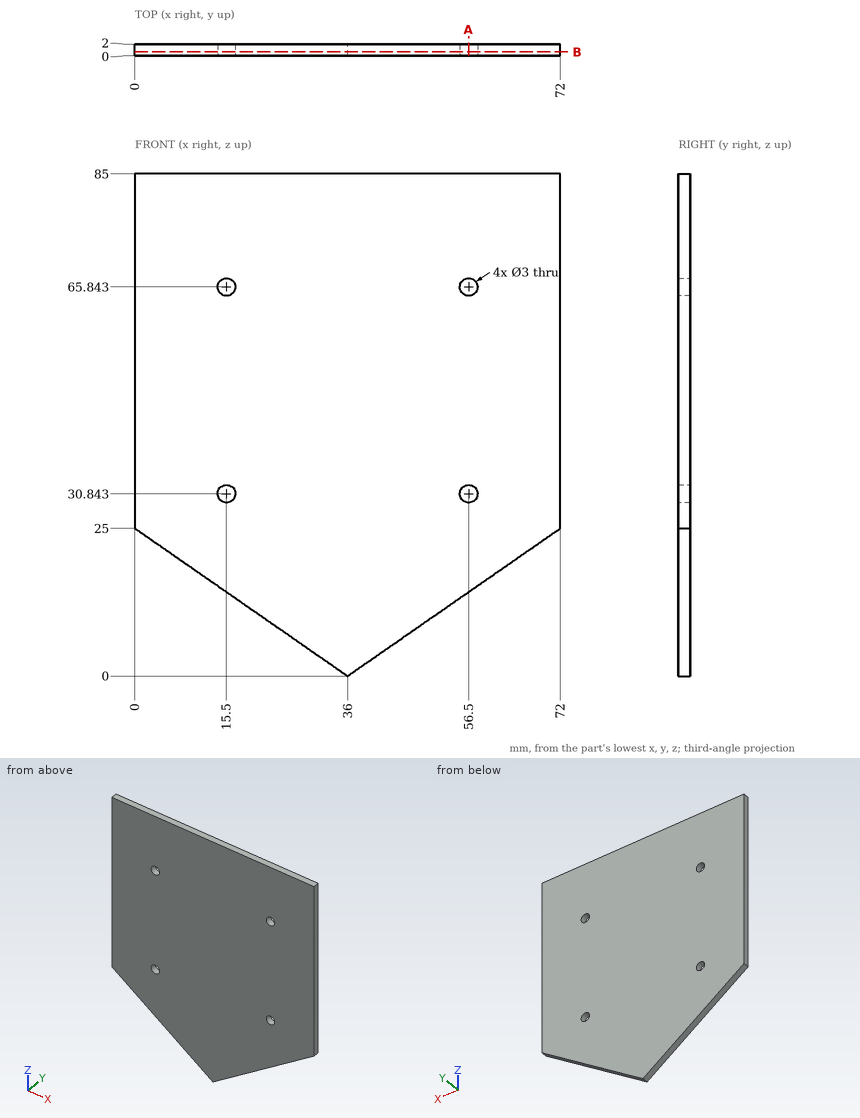
Design review of the part shown in the three views and the two pictorial views. Dimensions are in mm from the part's minimum x, y and z. Round coordinates to 2 decimals unless told otherwise and drop trailing zeros. Write each loop counter-clockwise with the first axis right and the second up, starting at its lowest first coordinate (ties: lowest second). Pieces come first, ordered by that corner, then holes. Notation, with made-up numbers: M -38,26 L -29,26 A24 cw -29,54 Z; hole C -28,21 d5. An arc over 180 degrees is marked long. One line per item, written item: value. Start each with the question number.
1. Clearance check with a flat-ended pin moving along its axis: P1, Ø4, axis at x = 15.5, z = 65.84, coming from the +Y side. State where the tip first meets the part, or that it passes through.
2. Take a section at B-B on y = 0.65. State the section outline as (x, z) points.
3. Take a section at A-A on x = 56.5. State the section outline as (y, z) points.
4. To check wall thickness, follow probe 1 along X at (y, z) = (1.6, 31); probe 2 along X at (y, z) = (1.35, 67) (1 decimal); probe 3 along X at (y, z) = (1.4, 16). State the ranges of each line that lie inside material, in increasing order. Write a range as from..to.
Computed:
1. P1: stops at y = 2
2. outline: M 0,25 L 36,0 L 72,25 L 72,85 L 0,85 Z; hole C 15.5,30.84 d3; hole C 15.5,65.84 d3; hole C 56.5,30.84 d3; hole C 56.5,65.84 d3
3. outline: M 0,14.24 L 2,14.24 L 2,29.34 L 0,29.34 Z; M 0,32.34 L 2,32.34 L 2,64.34 L 0,64.34 Z; M 0,67.34 L 2,67.34 L 2,85 L 0,85 Z
4. probe 1: x = 0..14.01, 16.99..55.01, 57.99..72
4. probe 2: x = 0..14.5, 16.5..55.5, 57.5..72
4. probe 3: x = 12.96..59.04
